from build123d import *

# Parameters (mm, degrees)
SKETCH1_R               = 19.05
BOSS_EXTRUDE1_DEPTH     = 12.7
SKETCH4_R               = 3.175
CUT_EXTRUDE2_DEPTH      = 13.7
CUT_EXTRUDE4_DEPTH      = 1
CUT_EXTRUDE4_DEPTH_BACK = 13.7
SKETCH7_R               = 6.35
BOSS_EXTRUDE2_DEPTH     = 6.35
CUT_EXTRUDE5_DEPTH      = 20.05


with BuildPart() as part:
    # Sketch1 → Boss-Extrude1 (new body)
    with BuildSketch(Plane.XY):
        Circle(SKETCH1_R)
    extrude(amount=BOSS_EXTRUDE1_DEPTH)

    # Sketch4 → Cut-Extrude2 (cut, through all)
    with BuildSketch(Plane(origin=(0, 0, 0), x_dir=(-1, 0, 0), z_dir=(0, 0, -1))):
        with Locations((0, 12.7)):
            Circle(SKETCH4_R)
        with Locations((0, -12.7)):
            Circle(SKETCH4_R)
    extrude(amount=-CUT_EXTRUDE2_DEPTH, mode=Mode.SUBTRACT)

    # Sketch6 → Cut-Extrude4 (cut, two sides)
    with BuildSketch(Plane.XY.offset(12.7)) as cut_extrude4_sk:
        with BuildLine():
            Line((1.546311471, 0.716838774), (0, 0.716838774))
            Line((0, 0.716838774), (-1.557372698, 0.716838774))
            ThreePointArc((-1.557372698, 0.716838774), (-0.005530614, -1.711645493), (1.546311471, 0.716838774))
        make_face()
    extrude(amount=CUT_EXTRUDE4_DEPTH, mode=Mode.SUBTRACT)
    extrude(cut_extrude4_sk.sketch, amount=-CUT_EXTRUDE4_DEPTH_BACK, mode=Mode.SUBTRACT)

    # Sketch7 → Boss-Extrude2 (add)
    with BuildSketch(Plane.XY.offset(12.7)):
        Circle(SKETCH7_R)
    extrude(amount=BOSS_EXTRUDE2_DEPTH)

    # Sketch8 → Cut-Extrude5 (cut, through all)
    with BuildSketch(Plane(origin=(0, 0, 0), x_dir=(-1, 0, 0), z_dir=(0, 0, -1))):
        with BuildLine():
            Line((-1.546311471, 0.716838774), (1.557372698, 0.716838774))
            ThreePointArc((1.557372698, 0.716838774), (0.005530614, -1.711645493), (-1.546311471, 0.716838774))
        make_face()
    extrude(amount=-CUT_EXTRUDE5_DEPTH, mode=Mode.SUBTRACT)


solid = part.part
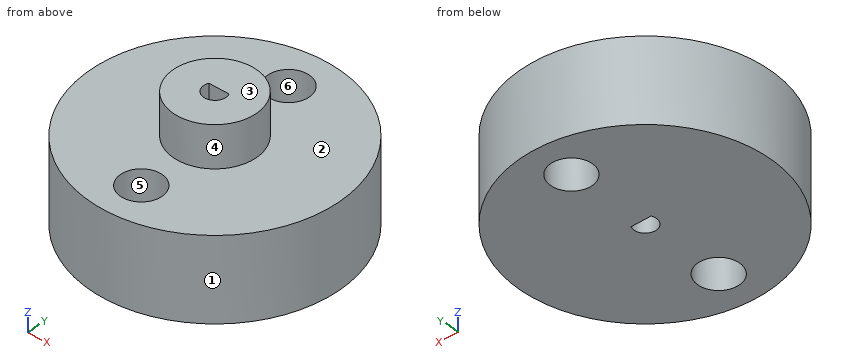
Here's how the part is built. I have some questions about the finished solid (model axes, mm). Face numbers are marked on the shaded views. A direction names the side the tool comes from. Round coordinates to 2 decimals unless told otherwise and drop trailing zeros. Loops run counter-clockwise (first coordinate to the right, second up) from the corner with the lowest first, then second, coordinate; pieces in that order, holes last. Notation, with made-up numbers: M 16.25,83.25 L 70.25,83.25 A9 ccw 70.25,91.25 Z; hole C 81.5,77.5 d10. An arc over 180 degrees is marked long. Write each question's results on one line, items separated by ' | '. Start each with the question number.
(1) On a 3-axis mill with a long thin cutter (end or side, diameter ignored), from which of +Z, -Z, +X, -X, +Y, -Y can I reach the whole of each face in a straight line? I mean the marked faces 1 and 2. Say none if no direction works.
(2) Thinking about a two-plate mould opening in X: for the marked faces 3, 4, 5 and 6, which applies, pulls with the +X half, pulls with the -X half, needs draft (parallel to the pull), parting line crosses it, or undercut?
(3) I want a section at B-B (y = 12.7). Please give me the cut outline in (x, z) (3 decimals).
(4) I want a section at D-D (z = 14.5). Please give me the cut outline in (x, y).
(5) I want a section at C-C (z = 1.5). Please give me the cut outline in (x, y) (3 decimals), then the cut area to 3 significant figures.
(6) Will these pins go through, and if not, where does the flat tip stop? P1, Ø5, axis at x = 2.5, z = 16.5, coming from the -Y side; P2, Ø12, axis at x = -3, y = 15, coming from the +Z side; P3, Ø2, axis at y = -8, z = 10, coming from the -X side.
(7) If I drill on probe 1 along Y at (x, z) = (0, 10) (3 decimals); probe 2 along Z at (x, y) = (6, 6); probe 3 along X at (y, z) = (-15, 12.5), over which ranges is the centre line in solid material (lowest first)? Write a range as from..to.
(8) I want a section at A-A (x = 0). Please give me the cut outline in (y, z) (3 decimals).
Solved:
1) face 1: +Z, -Z | face 2: +Z
2) face 3: needs draft | face 4: parting line crosses it | face 5: undercut | face 6: undercut
3) outline: M -14.199,0 L -3.175,0 L -3.175,12.7 L -14.199,12.7 Z; M 3.175,0 L 14.199,0 L 14.199,12.7 L 3.175,12.7 Z
4) outline: C 0,0 d12.7; hole M -1.56,0.72 A1.71 ccw long 1.55,0.72 Z
5) outline: C 0,0 d38.1; hole C 0,-12.7 d6.35; hole C 0,12.7 d6.35; hole M -1.557,0.717 A1.71 ccw long 1.546,0.717 Z | area: 1,070 mm²
6) P1: stops at y = -6.35 | P2: stops at z = 12.7 | P3: stops at x = -17.72
7) probe 1: y = -19.05..-15.875, -9.525..-1.712, 0.717..9.525, 15.875..19.05 | probe 2: z = 0..12.7 | probe 3: x = -11.74..-2.19, 2.19..11.74
8) outline: M -19.05,0 L -15.875,0 L -15.875,12.7 L -19.05,12.7 Z; M -9.525,0 L -1.712,0 L -1.712,19.05 L -6.35,19.05 L -6.35,12.7 L -9.525,12.7 Z; M 0.717,0 L 9.525,0 L 9.525,12.7 L 6.35,12.7 L 6.35,19.05 L 0.717,19.05 Z; M 15.875,0 L 19.05,0 L 19.05,12.7 L 15.875,12.7 Z
